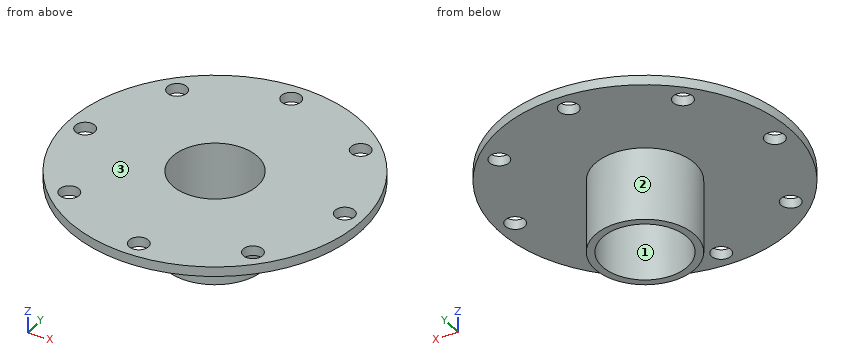
Autodesk Inventor part; units mm, degrees
ref_plane "YZ Plane" through (0, 0, 0) normal (1, 0, 0) x (0, 1, 0)
ref_plane "XZ Plane" through (0, 0, 0) normal (0, 1, 0) x (-1, 0, 0)
ref_plane "XY Plane" through (0, 0, 0) normal (0, 0, 1) x (1, 0, 0)
sketch "Boceto1" plane through (0, 0, 0) normal (0, 0, 1) x (1, 0, 0)
  circle A0 centre (0, 0) radius 60
  circle A1 centre (0, 0) radius 48.5 construction
  circle A2 centre (0, 0) radius 52.5 construction
  line L0 (0, -61.2439) -> (0, 59.6068) construction
  line L1 (-77.557, 0) -> (94.8903, 0) construction
  circle A3 centre (0, 52.5) radius 4
  circle A4 centre (-37.1231, 37.1231) radius 4
  circle A5 centre (-52.5, 0) radius 4
  circle A6 centre (-37.1231, -37.1231) radius 4
  circle A7 centre (0, -52.5) radius 4
  circle A8 centre (37.1231, -37.1231) radius 4
  circle A9 centre (52.5, 0) radius 4
  circle A10 centre (37.1231, 37.1231) radius 4
  dimension "d2" = 105
  dimension "d0" = 120
  dimension "d1" = 97
  dimension "d3" = 8
  dimension "d6" = 360
extrude "Extrusión1" add sketch "Boceto1" along normal blind 4
sketch "Boceto2" plane through (0, 0, 0) normal (0, 0, -1) x (-1, 0, 0)
  circle A0 centre (0, 0) radius 20.5
  dimension "d10" = 41
extrude "Extrusión2" add sketch "Boceto2" along normal blind 30
sketch "Boceto3" plane through (0, 0, -30) normal (0, 0, -1) x (-1, 0, 0)
  circle A0 centre (0, 0) radius 17.5
  dimension "d13" = 35
extrude "Extrusión3" cut sketch "Boceto3" against normal blind 35
properties part number "CESTO MEDIDOR ESPORAS"
Can you work these out from the model? Positions are in its coordinate system, mm. Face numbers are marked on the shaded views. Round coordinates to 2 decimals unless told otherwise and drop trailing zeros. Order: outer loops, then holes, each group sorted by start corner. A loop starts at its lowest first (then second) coordinate and runs counter-clockwise, first axis right, second up. Notation, with made-up numbers: (18, -1.75) -> (32, -1.75) arc R32 ccw to (32, 30.25) -> close; hole circle Ø5 at (40.25, 40). An arc over 180 degrees is marked (long way). Write each question's results on one line, items separated by ' | '. Start each with the question number.
Item 1: Please list where these lines run through material, in increasing order: L1, parallel to Y at x = 0, z = 1; L2, parallel to Y at x = -33.5, z = 2.5; L3, parallel to X at y = -9, z = -15.5.
Item 2: If we section it at A-A, the plane y = 0: Write out the boundary of the cut face in (x, z).
Item 3: If we section it at C-C, the plane x = 52.5: Write out the boundary of the cut face in (y, z).
Item 4: Thinking about a two-plate mould opening in X: for the marked faces 1, 2 and 3, which applies, +X half, -X half, draft (parallel to the pull), parting line (faces both ways), or undercut?
Item 5: If we section it at D-D, the plane y = -14.5: Write out the boundary of the cut face in (x, z).
Item 6: Will these pins go through, and if not, where does the flat tip stop? pin 1 (6 mm diameter, centred on x = 12, z = -24, fed in from +Y); pin 2 (10.5 mm diameter, centred on x = -37.12, y = 37.12, fed in from +Z); pin 3 (2 mm diameter, centred on x = -34.5, y = 41.5, fed in from -Z); pin 4 (6 mm diameter, centred on y = 0, z = -20.5, fed in from +X).
Results:
1) L1: y = -60 to -56.5, -48.5 to -17.5, 17.5 to 48.5, 56.5 to 60 | L2: y = -49.78 to -38.82, -35.43 to 35.43, 38.82 to 49.78 | L3: x = -18.42 to -15.01, 15.01 to 18.42
2) outline: (-60, 0) -> (-56.5, 0) -> (-56.5, 4) -> (-60, 4) -> close; (-48.5, 0) -> (-20.5, 0) -> (-20.5, -30) -> (-17.5, -30) -> (-17.5, 4) -> (-48.5, 4) -> close; (17.5, -30) -> (20.5, -30) -> (20.5, 0) -> (48.5, 0) -> (48.5, 4) -> (17.5, 4) -> close; (56.5, 0) -> (60, 0) -> (60, 4) -> (56.5, 4) -> close
3) outline: (-29.05, 0) -> (-4, 0) -> (-4, 4) -> (-29.05, 4) -> close; (4, 0) -> (29.05, 0) -> (29.05, 4) -> (4, 4) -> close
4) face 1: undercut | face 2: parting line | face 3: draft
5) outline: (-58.22, 0) -> (-14.49, 0) -> (-14.49, -30) -> (-9.8, -30) -> (-9.8, 4) -> (-58.22, 4) -> close; (9.8, -30) -> (14.49, -30) -> (14.49, 0) -> (58.22, 0) -> (58.22, 4) -> (9.8, 4) -> close
6) pin 1: stops at y = 18.42 | pin 2: stops at z = 4 | pin 3: stops at z = 0 | pin 4: stops at x = 20.5
